The listing builds one solid part. Answer for the finished solid, in the listing's coordinates (mm). Face numbers are marked on the shaded views. A direction names the side the tool comes from. Give positions to 0.01 mm unless a question says otherwise; leave off trailing zeros. Write each loop counter-clockwise with the first axis right and the second up, starting at its lowest first coordinate (ties: lowest second). Pieces come first, ordered by that corner, then holes.
```python
from build123d import *

# Parameters (mm, degrees)
BOSS_EXTRUDE2_DEPTH     = 4
FILLET1_R               = 0.5
FILLET2_R               = 0.5
CUT_EXTRUDE1_DEPTH      = 35.96700514
CUT_EXTRUDE1_DEPTH_BACK = 35.96700514
SKETCH4_R               = 2


with BuildPart() as part:
    # Sketch3 → Boss-Extrude2 (new body)
    with BuildSketch(Plane.XY):
        with BuildLine():
            ThreePointArc((-10.014736402, 19.376191891), (-9.990551511, 18.103554733), (-10.776995598, 17.102707121))
            ThreePointArc((-10.776995598, 17.102707121), (-20.215, 0), (-10.776995598, -17.102707121))
            ThreePointArc((-10.776995598, -17.102707121), (-9.990551511, -18.103554733), (-10.014736402, -19.376191891))
            ThreePointArc((-10.014736402, -19.376191891), (-10.36939918, -19.711941674), (-10.776995598, -19.98097469))
            ThreePointArc((-10.776995598, -19.98097469), (-12.938385888, -21.864089687), (-14.088666538, -24.48984377))
            ThreePointArc((-14.088666538, -24.48984377), (-13.85696402, -25.752415366), (-12.828666538, -26.520775556))
            ThreePointArc((-12.828666538, -26.520775556), (-6.472322707, -27.815519537), (0, -28.249694219))
            ThreePointArc((0, -28.249694219), (6.472322707, -27.815519537), (12.828666538, -26.520775556))
            ThreePointArc((12.828666538, -26.520775556), (13.85696402, -25.752415366), (14.088666538, -24.48984377))
            ThreePointArc((14.088666538, -24.48984377), (12.938385888, -21.864089687), (10.776995598, -19.98097469))
            ThreePointArc((10.776995598, -19.98097469), (10.36939918, -19.711941674), (10.014736402, -19.376191891))
            ThreePointArc((10.014736402, -19.376191891), (9.990551511, -18.103554733), (10.776995598, -17.102707121))
            ThreePointArc((10.776995598, -17.102707121), (20.215, 0), (10.776995598, 17.102707121))
            ThreePointArc((10.776995598, 17.102707121), (9.990551511, 18.103554733), (10.014736402, 19.376191891))
            ThreePointArc((10.014736402, 19.376191891), (10.36939918, 19.711941674), (10.776995598, 19.98097469))
            ThreePointArc((10.776995598, 19.98097469), (12.938385888, 21.864089687), (14.088666538, 24.48984377))
            ThreePointArc((14.088666538, 24.48984377), (13.85696402, 25.752415366), (12.828666538, 26.520775556))
            ThreePointArc((12.828666538, 26.520775556), (6.472322707, 27.815519537), (0, 28.249694219))
            ThreePointArc((0, 28.249694219), (-6.472322707, 27.815519537), (-12.828666538, 26.520775556))
            ThreePointArc((-12.828666538, 26.520775556), (-13.85696402, 25.752415366), (-14.088666538, 24.48984377))
            ThreePointArc((-14.088666538, 24.48984377), (-12.938385888, 21.864089687), (-10.776995598, 19.98097469))
            ThreePointArc((-10.776995598, 19.98097469), (-10.36939918, 19.711941674), (-10.014736402, 19.376191891))
        make_face()
        with BuildLine():
            Line((-12.828666538, -1.774676079), (-12.828666538, 1.774676079))
            Line((-12.828666538, 1.774676079), (-14.088666538, 1.774676079))
            ThreePointArc((-14.088666538, 1.774676079), (0, 14.2), (14.088666538, 1.774676079))
            Line((14.088666538, 1.774676079), (12.828666538, 1.774676079))
            Line((12.828666538, 1.774676079), (12.828666538, -1.774676079))
            Line((12.828666538, -1.774676079), (14.088666538, -1.774676079))
            ThreePointArc((14.088666538, -1.774676079), (0, -14.2), (-14.088666538, -1.774676079))
            Line((-14.088666538, -1.774676079), (-12.828666538, -1.774676079))
        make_face(mode=Mode.SUBTRACT)
    extrude(amount=BOSS_EXTRUDE2_DEPTH)

    # Fillet1
    fillet1_edges = [part.edges().sort_by_distance(p)[0] for p in [
        (-12.828666538, 1.774676079, 2),
        (-12.828666538, -1.774676079, 2),
        (12.828666538, -1.774676079, 2),
        (12.828666538, 1.774676079, 2),
    ]]
    fillet(fillet1_edges, radius=FILLET1_R)

    # Fillet2
    fillet2_edges = [part.edges().sort_by_distance(p)[0] for p in [
        (-14.088666538, 1.774676079, 2),
        (-14.088666538, -1.774676079, 2),
        (14.088666538, -1.774676079, 2),
        (14.088666538, 1.774676079, 2),
    ]]
    fillet(fillet2_edges, radius=FILLET2_R)

    # Sketch4 → Cut-Extrude1 (cut, two sides: drawn at the far end of the back side and taken through both)
    with BuildSketch(Plane.XY.offset(4).offset(-CUT_EXTRUDE1_DEPTH_BACK)):
        with Locations((0, 23.749694219)):
            Circle(SKETCH4_R)
        with Locations(Location((0, -23.749694219, 0), (0, 0, 180))):
            Circle(SKETCH4_R)
    extrude(amount=CUT_EXTRUDE1_DEPTH + CUT_EXTRUDE1_DEPTH_BACK, mode=Mode.SUBTRACT)


solid = part.part
```
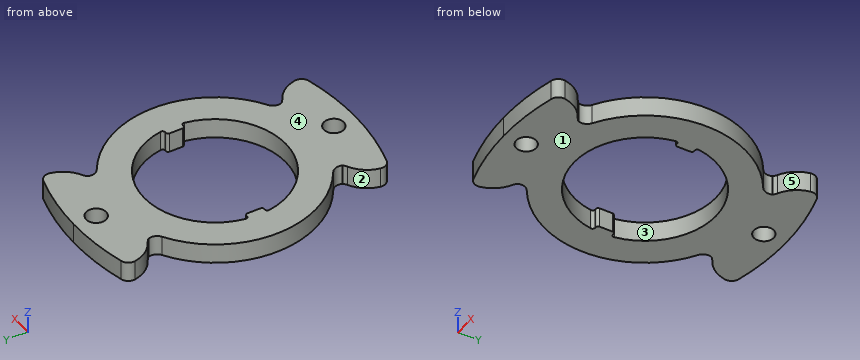
Item 1: Which of the six approach directions +Z, -Z, +X, -X, +Y, -Y give full straight-line access (tool end or side, diameter ignored) to the marked faces 1, 2 and 3?
Conclusion:
face 1: -Z, +X, -X, +Y, -Y
face 2: +Z, -Z, -X
face 3: +Z, -Z
Item 2: Consider probe 1 along Y at (x, z) = (-10.5, 1.4); probe 2 along Y at (x, z) = (11.5, 1.45); probe 3 along X at (y, z) = (6, 2.55). Determine where each line is inside the solid, lowest interval first.
Conclusion:
probe 1: y = -27.1 to -19.81, -17.32 to -9.56, 9.56 to 17.32, 19.81 to 27.1
probe 2: y = -26.87 to -20.44, -16.63 to -8.33, 8.33 to 16.63, 20.44 to 26.87
probe 3: x = -19.3 to -12.87, 12.87 to 19.3
Item 3: A cutting plane is placed at B-B, the plane y = 6. Give the vertices of the cut face in (x, z).
Conclusion:
outline: (-19.3, 0) - (-12.87, 0) - (-12.87, 4) - (-19.3, 4) - close; (12.87, 0) - (19.3, 0) - (19.3, 4) - (12.87, 4) - close
Item 4: Determine the mould class of the marked faces 4 and 5 for opening direction Y: pulls with the +Y half, pulls with the -Y half, needs draft (parallel to the pull), parting line crosses it, or undercut.
Conclusion:
face 4: needs draft
face 5: undercut
Item 5: A cutting plane is placed at C-C, the plane z = 2.6. Count the separate pieces of the cut face and the enclosed holes in it, plus the area to 3 significant figures.
Conclusion:
separate pieces: 1
enclosed holes: 3
area: 1,070 mm2
Item 6: A cutting plane is placed at A-A, the plane x = 8.5. Give the vertices of the cut face in (y, z).
Conclusion:
outline: (-27.5, 0) - (-11.37, 0) - (-11.37, 4) - (-27.5, 4) - close; (11.37, 0) - (27.5, 0) - (27.5, 4) - (11.37, 4) - close
Item 7: A cutting plane is placed at D-D, the plane y = 15.5. Give the vertices of the cut face in (x, z).
Conclusion:
outline: (-12.98, 0) - (12.98, 0) - (12.98, 4) - (-12.98, 4) - close
Item 8: Each of these flat-tipped pins is pushed along its axis until it touches: P1, Ø1.5, axis at y = 5.5, z = 2.5, coming from the -X side; P2, Ø2, axis at y = -3, z = 1.5, coming from the -X side; P3, Ø3.5, axis at x = 0, y = -23.75, coming from the -Z side; P4, Ø1, axis at x = 14, z = 3, coming from the +Y side. Where does it stop, or does it pass through?
Conclusion:
P1: stops at x = -19.65
P2: stops at x = -20.12
P3: passes through
P4: stops at y = 26.17
